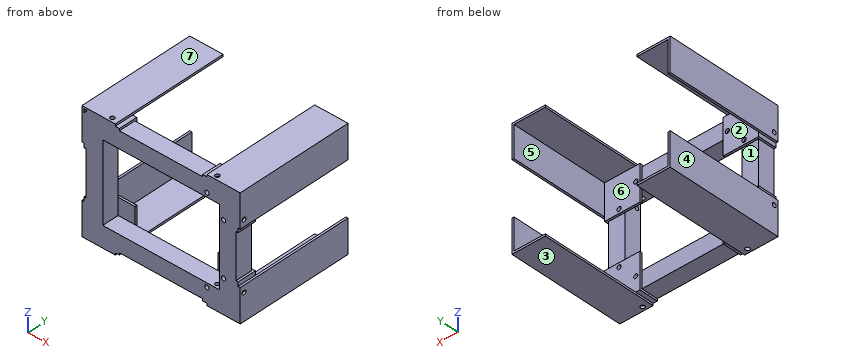
from build123d import *
from build123d.topology import SkipClean

# Parameters (mm, degrees)
SKETCH2_W             = 25.4
SKETCH2_H             = 119.38
BOSS_EXTRUDE1_DEPTH   = 25.4
SKETCH8_W             = 50.8
SKETCH8_H             = 3.175
BOSS_EXTRUDE9_DEPTH   = 25.4
SKETCH11_W            = 53.975
SKETCH11_H            = 53.975
BOSS_EXTRUDE12_DEPTH  = 3.175
CHAMFER3_SIZE         = 5.08
SKETCH10_W            = 3.175
SKETCH10_H            = 47.625
BOSS_EXTRUDE11_DEPTH  = 177.8
SKETCH13_R            = 3.175
CUT_EXTRUDE3_DEPTH    = 31.75
SKETCH14_R            = 3.175
CUT_EXTRUDE4_DEPTH    = 28.575
SKETCH16_R            = 3.175
CUT_EXTRUDE5_DEPTH    = 31.75
MIRROR71_START        = -1
MIRROR71_OUTLINE_R    = 3.175
MIRROR71_DEPTH        = 26.4
MIRROR71_2_DEPTH      = 177.8
MIRROR71_START_2      = 25.4
MIRROR71_3_OUTLINE_R  = 3.175
MIRROR71_3_DEPTH      = 3.175
MIRROR71_START_3      = 9.525
MIRROR71_4_OUTLINE_R  = 3.175
MIRROR71_4_DEPTH      = 15.875
MIRROR71_5_OUTLINE_R  = 3.175
MIRROR71_5_DEPTH      = 3.1749999
MIRROR71_START_4      = 2.6969085
MIRROR71_6_OUTLINE_R  = 3.175
MIRROR71_6_DEPTH      = 17.145
MIRROR71_START_5      = -85.09
MIRROR71_7_OUTLINE_W  = 3.175
MIRROR71_7_OUTLINE_H  = 6.3500001
MIRROR71_7_OUTLINE_R  = 3.175
MIRROR71_7_DEPTH      = 25.4
MIRROR71_START_6      = 59.69
MIRROR71_8_DEPTH      = 28.575
MIRROR71_START_7      = -88.265
MIRROR71_9_DEPTH      = 3.175
MIRROR71_START_8      = 85.09
MIRROR71_10_DEPTH     = 3.175
MIRROR71_START_9      = -91.896565
MIRROR71_11_OUTLINE_W = 6.3500001
MIRROR71_11_OUTLINE_H = 25.4
MIRROR71_11_DEPTH     = 155.396565
MIRROR71_START_10     = 88.9
MIRROR71_12_DEPTH     = 28.575
MIRROR71_START_11     = -114.3
MIRROR71_13_OUTLINE_R = 3.175
MIRROR71_13_DEPTH     = 25.4
MIRROR71_START_12     = 114.3
MIRROR71_14_DEPTH     = 3.175
MIRROR71_START_13     = -92
MIRROR71_15_OUTLINE_R = 3.175
MIRROR71_15_DEPTH     = 184
MIRROR71_16_OUTLINE_R = 3.175
MIRROR71_16_DEPTH     = 33.1


with BuildPart() as part:
    # Sketch2 → Boss-Extrude1 (new body)
    with BuildSketch(Plane(origin=(0, 0, 0), x_dir=(1, 0, 0), z_dir=(0, 1, 0))):
        Polygon((114.3, -59.69), (88.9, -59.69), (-88.9, -59.69), (-114.3, -59.69), (-114.3, -85.09), (114.3, -85.09), align=None)
        with Locations((101.6, 0)):
            Rectangle(SKETCH2_W, SKETCH2_H)
        Polygon((-88.9, 59.69), (88.9, 59.69), (114.3, 59.69), (114.3, 85.09), (-114.3, 85.09), (-114.3, 59.69), align=None)
        with Locations((-101.6, 0)):
            Rectangle(SKETCH2_W, SKETCH2_H)
    boss_extrude1 = extrude(amount=BOSS_EXTRUDE1_DEPTH)

    # Sketch8 → Boss-Extrude9 (add)
    with BuildSketch(Plane(origin=(0, 25.4, 0), x_dir=(1, 0, 0), z_dir=(0, 1, 0))):
        with Locations((-88.9, -86.6775)):
            Rectangle(SKETCH8_W, SKETCH8_H)
        Polygon((-114.3, -88.265), (-114.3, -85.09), (-114.3, -34.29), (-117.475, -34.29), (-117.475, -88.265), align=None)
    boss_extrude9 = extrude(amount=-BOSS_EXTRUDE9_DEPTH)

    # Sketch11 → Boss-Extrude12 (add)
    with BuildSketch(Plane(origin=(0, 25.4, 0), x_dir=(1, 0, 0), z_dir=(0, 1, 0))):
        with Locations((-90.4875, -61.2775)):
            Rectangle(SKETCH11_W, SKETCH11_H)
    boss_extrude12 = extrude(amount=BOSS_EXTRUDE12_DEPTH)

    # Chamfer3
    chamfer3_edges = [part.edges().sort_by_distance(p)[0] for p in [
        (-117.475, 14.2875, 88.265),
    ]]
    chamfer(chamfer3_edges, length=CHAMFER3_SIZE)

    # Sketch10 → Boss-Extrude11 (add)
    with BuildSketch(Plane(origin=(0, 0, 0), x_dir=(-1, 0, 0), z_dir=(0, -1, 0))):
        with Locations((119.0625, -64.4525)):
            Rectangle(SKETCH10_W, SKETCH10_H)
        Polygon((120.65, -88.265), (117.475, -88.265), (69.85, -88.265), (69.85, -91.44), (120.65, -91.44), align=None)
    boss_extrude11 = extrude(amount=-BOSS_EXTRUDE11_DEPTH)

    # Sketch13 → Cut-Extrude3 (cut)
    with BuildSketch(Plane.XY.offset(91.44)):
        with Locations((-80.01, 6.35)):
            Circle(SKETCH13_R)
    cut_extrude3 = extrude(amount=-CUT_EXTRUDE3_DEPTH, mode=Mode.SUBTRACT)

    # Sketch14 → Cut-Extrude4 (cut)
    with BuildSketch(Plane(origin=(0, 28.575, 0), x_dir=(1, 0, 0), z_dir=(0, 1, 0))):
        with Locations(Location((-69.85, -66.04, 0), (0, 0, 270))):
            Circle(SKETCH14_R)
        with Locations(Location((-95.25, -40.64, 0), (0, 0, 270))):
            Circle(SKETCH14_R)
    cut_extrude4 = extrude(amount=-CUT_EXTRUDE4_DEPTH, mode=Mode.SUBTRACT)

    # Sketch16 → Cut-Extrude5 (cut)
    with BuildSketch(Plane.ZY.offset(120.65)):
        with Locations((50.8, 6.35)):
            Circle(SKETCH16_R)
    cut_extrude5 = extrude(amount=-CUT_EXTRUDE5_DEPTH, mode=Mode.SUBTRACT)

    # Mirror70: Boss-Extrude1, Boss-Extrude9, Boss-Extrude12, Boss-Extrude11, Cut-Extrude3, Cut-Extrude4, Cut-Extrude5 across plane
    add(boss_extrude1.mirror(Plane.XY))
    add(boss_extrude9.mirror(Plane.XY))
    add(boss_extrude12.mirror(Plane.XY))
    add(boss_extrude11.mirror(Plane.XY))
    add(cut_extrude3.mirror(Plane.XY), mode=Mode.SUBTRACT)
    add(cut_extrude4.mirror(Plane.XY), mode=Mode.SUBTRACT)
    add(cut_extrude5.mirror(Plane.XY), mode=Mode.SUBTRACT)

    # Mirror71: read off the stored shape, not the designer's step
    # Mirror71 outline → Mirror71 (cut)
    with BuildSketch(Plane(origin=(0, 0, 0), x_dir=(1, 0, 0), z_dir=(0, 1, 0)).offset(MIRROR71_START)):
        with Locations((69.85, 66.04)):
            Circle(MIRROR71_OUTLINE_R)
        with Locations((95.25, 40.64)):
            Circle(MIRROR71_OUTLINE_R)
        with Locations((69.85, -66.04)):
            Circle(MIRROR71_OUTLINE_R)
        with Locations((95.25, -40.64)):
            Circle(MIRROR71_OUTLINE_R)
    extrude(amount=MIRROR71_DEPTH, mode=Mode.SUBTRACT)



with BuildPart() as body_2:
    # Mirror71 2 outline → Mirror71 2 (new body)
    with BuildSketch(Plane(origin=(0, 0, 0), x_dir=(1, 0, 0), z_dir=(0, 1, 0))):
        Polygon((117.475, -88.265), (69.85, -88.265), (69.85, -91.44), (120.65, -91.44), (120.65, -40.64), (117.475, -40.64), align=None)
        Polygon((117.475, 88.265), (117.475, 40.64), (120.65, 40.64), (120.65, 91.44), (69.85, 91.44), (69.85, 88.265), align=None)
    extrude(amount=MIRROR71_2_DEPTH)


with BuildPart() as part_1:
    add(part.part)

    add(body_2.part)  # Mirror71 3 merges body 2
    # Mirror71 3 outline → Mirror71 3 (add)
    # profile 1 of 2: a face of its own
    with BuildSketch(Plane(origin=(0, 0, 0), x_dir=(1, 0, 0), z_dir=(0, 1, 0)).offset(MIRROR71_START_2)):
        Polygon((63.5, -88.265), (117.475, -88.265), (117.475, -34.29), (88.9, -34.29), (63.5, -34.29), align=None)
        with Locations((95.25, -40.64)):
            Circle(MIRROR71_3_OUTLINE_R, mode=Mode.SUBTRACT)
        with Locations((69.85, -66.04)):
            Circle(MIRROR71_3_OUTLINE_R, mode=Mode.SUBTRACT)
    # profile 2 of 2: a face of its own
    with BuildSketch(Plane(origin=(0, 0, 0), x_dir=(1, 0, 0), z_dir=(0, 1, 0)).offset(MIRROR71_START_2)):
        Polygon((63.5, 34.29), (88.9, 34.29), (117.475, 34.29), (117.475, 88.265), (63.5, 88.265), align=None)
        with Locations((95.25, 40.64)):
            Circle(MIRROR71_3_OUTLINE_R, mode=Mode.SUBTRACT)
        with Locations((69.85, 66.04)):
            Circle(MIRROR71_3_OUTLINE_R, mode=Mode.SUBTRACT)
    extrude(amount=MIRROR71_3_DEPTH)

    # Mirror71 4 outline → Mirror71 4 (add)
    with BuildSketch(Plane(origin=(0, 0, 0), x_dir=(1, 0, 0), z_dir=(0, 1, 0)).offset(MIRROR71_START_3)):
        Polygon((63.5, -88.265), (117.475, -88.265), (117.475, -34.29), (114.3, -34.29), (114.3, -85.09), (63.5, -85.09), align=None)
        Polygon((114.3, 85.09), (114.3, 34.29), (117.475, 34.29), (117.475, 88.265), (63.5, 88.265), (63.5, 85.09), align=None)
        with Locations((-69.85, 66.04)):
            Circle(MIRROR71_4_OUTLINE_R)
        with Locations((-95.25, 40.64)):
            Circle(MIRROR71_4_OUTLINE_R)
    extrude(amount=MIRROR71_4_DEPTH)

    # Mirror71 5 outline → Mirror71 5 (add)
    with BuildSketch(Plane(origin=(0, 0, 0), x_dir=(1, 0, 0), z_dir=(0, 1, 0))):
        Polygon((63.5, -88.265), (117.475, -88.265), (117.475, -34.29), (114.3, -34.29), (114.3, -85.09), (63.5, -85.09), align=None)
        Polygon((114.3, 85.09), (114.3, 34.29), (117.475, 34.29), (117.475, 88.265), (63.5, 88.265), (63.5, 85.09), align=None)
        with Locations((-69.85, 66.04)):
            Circle(MIRROR71_5_OUTLINE_R)
        with Locations((-95.25, 40.64)):
            Circle(MIRROR71_5_OUTLINE_R)
    extrude(amount=MIRROR71_5_DEPTH)

    # Mirror71 6 outline → Mirror71 6 (add)
    with BuildSketch(Plane(origin=(0, 0, 0), x_dir=(1, 0, 0), z_dir=(0, 1, 0)).offset(MIRROR71_START_4)):
        with Locations((-69.85, 66.04)):
            Circle(MIRROR71_6_OUTLINE_R)
        with Locations((-95.25, 40.64)):
            Circle(MIRROR71_6_OUTLINE_R)
    extrude(amount=MIRROR71_6_DEPTH)

    # Mirror71 7 outline → Mirror71 7 (add)
    with BuildSketch(Plane.XY.offset(MIRROR71_START_5)):
        with Locations((115.8875, 6.34999995)):
            Rectangle(MIRROR71_7_OUTLINE_W, MIRROR71_7_OUTLINE_H)
        with Locations((-80.01, 6.35)):
            Circle(MIRROR71_7_OUTLINE_R)
    extrude(amount=MIRROR71_7_DEPTH)

    # Mirror71 8 outline → Mirror71 8 (add)
    with BuildSketch(Plane.XY.offset(MIRROR71_START_6)):
        with BuildLine():
            ThreePointArc((80.01, 9.525), (83.185, 6.35), (80.01, 3.175))
            Line((80.01, 3.175), (117.475, 3.1749999))
            Line((117.475, 3.1749999), (117.475, 9.525))
            Line((117.475, 9.525), (80.01, 9.525))
        make_face()
    extrude(amount=MIRROR71_8_DEPTH)

    # Mirror71 9 outline → Mirror71 9 (add)
    with BuildSketch(Plane.XY.offset(MIRROR71_START_7)):
        with BuildLine():
            ThreePointArc((80.01, 9.525), (83.185, 6.35), (80.01, 3.175))
            Line((80.01, 3.175), (117.475, 3.1749999))
            Line((117.475, 3.1749999), (117.475, 9.525))
            Line((117.475, 9.525), (80.01, 9.525))
        make_face()
        with BuildLine():
            ThreePointArc((80.01, 3.175), (76.835, 6.35), (80.01, 9.525))
            Line((80.01, 9.525), (63.5, 9.525))
            Line((63.5, 9.525), (63.5, 3.1749999))
            Line((63.5, 3.1749999), (80.01, 3.175))
        make_face()
    extrude(amount=MIRROR71_9_DEPTH)

    # Mirror71 10 outline → Mirror71 10 (add)
    with BuildSketch(Plane.XY.offset(MIRROR71_START_8)):
        with BuildLine():
            ThreePointArc((80.01, 3.175), (76.835, 6.35), (80.01, 9.525))
            Line((80.01, 9.525), (63.5, 9.525))
            Line((63.5, 9.525), (63.5, 3.1749999))
            Line((63.5, 3.1749999), (80.01, 3.175))
        make_face()
    extrude(amount=MIRROR71_10_DEPTH)

    # Mirror71 11 outline → Mirror71 11 (add)
    with BuildSketch(Plane.YZ.offset(MIRROR71_START_9)):
        with Locations((6.34999995, -72.39)):
            Rectangle(MIRROR71_11_OUTLINE_W, MIRROR71_11_OUTLINE_H)
    extrude(amount=MIRROR71_11_DEPTH)

    # Mirror71 12 outline → Mirror71 12 (add)
    with BuildSketch(Plane.YZ.offset(MIRROR71_START_10)):
        with BuildLine():
            ThreePointArc((9.525, -50.8), (6.35, -53.975), (3.175, -50.8))
            Line((3.175, -50.8), (3.1749999, -88.265))
            Line((3.1749999, -88.265), (9.525, -88.265))
            Line((9.525, -88.265), (9.525, -50.8))
        make_face()
        with BuildLine():
            ThreePointArc((3.175, 50.8), (6.35, 53.975), (9.525, 50.8))
            Line((9.525, 50.8), (9.525, 88.265))
            Line((9.525, 88.265), (3.1749999, 88.265))
            Line((3.1749999, 88.265), (3.175, 50.8))
        make_face()
    extrude(amount=MIRROR71_12_DEPTH)

    # Mirror71 13 outline → Mirror71 13 (add)
    with BuildSketch(Plane.YZ.offset(MIRROR71_START_11)):
        with Locations((6.35, -50.8)):
            Circle(MIRROR71_13_OUTLINE_R)
    extrude(amount=MIRROR71_13_DEPTH)

    # Mirror71 14 outline → Mirror71 14 (add)
    with BuildSketch(Plane.YZ.offset(MIRROR71_START_12)):
        with BuildLine():
            ThreePointArc((3.175, -50.8), (6.35, -47.625), (9.525, -50.8))
            Line((9.525, -50.8), (9.525, -34.29))
            Line((9.525, -34.29), (3.1749999, -34.29))
            Line((3.1749999, -34.29), (3.175, -50.8))
        make_face()
        with BuildLine():
            Line((9.525, 34.29), (9.525, 50.8))
            ThreePointArc((9.525, 50.8), (6.35, 47.625), (3.175, 50.8))
            Line((3.175, 50.8), (3.1749999, 34.29))
            Line((3.1749999, 34.29), (9.525, 34.29))
        make_face()
    extrude(amount=MIRROR71_14_DEPTH)

    # Mirror71 15 outline → Mirror71 15 (cut)
    with SkipClean():  # the faces are left unmerged after this step: merging them gives an invalid solid
        with BuildSketch(Plane.XY.offset(MIRROR71_START_13)):
            with Locations((80.01, 6.35)):
                Circle(MIRROR71_15_OUTLINE_R)
        extrude(amount=MIRROR71_15_DEPTH, mode=Mode.SUBTRACT)

    # Mirror71 16 outline → Mirror71 16 (cut)
    with SkipClean():  # the faces are left unmerged after this step: merging them gives an invalid solid
        with BuildSketch(Plane.YZ.offset(MIRROR71_START_10)):
            with Locations((6.35, -50.8)):
                Circle(MIRROR71_16_OUTLINE_R)
            with Locations((6.35, 50.8)):
                Circle(MIRROR71_16_OUTLINE_R)
        extrude(amount=MIRROR71_16_DEPTH, mode=Mode.SUBTRACT)


solid = part_1.part
For this review, take the finished solid that the model builds, in its own axes (mm). Face numbers are marked on the shaded views. A direction names the side the tool comes from. Give positions to 0.01 mm unless a question says otherwise; leave off trailing zeros. Loops run counter-clockwise (first coordinate to the right, second up) from the corner with the lowest first, then second, coordinate; pieces in that order, holes last.
Item 1: Take a section at B-B, the plane y = 56. State the section outline as (x, z) points (3 decimals).
Item 2: Take a section at D-D, the plane x = -95.25. State the section outline as (y, z) points (3 decimals).
Item 3: Take a section at C-C, the plane z = -27. State the section outline as (x, y) points, and give its area (3 significant figures).
Item 4: Draft analysis for pull direction X (two halves, no side actions). For the marked faces 4, 5, 6 and 7, state which applies: +X half, -X half, draft (parallel to the pull), parting line (faces both ways), or undercut.
Item 5: Tool access review of the marked faces 1, 2 and 3: name each direction out of +Z, -Z, +X, -X, +Y, -Y from which nothing blocks a thin tool from reaching the whole face with its end or side.
Item 6: Take a section at A-A, the plane x = 53.5. State the section outline as (y, z) points.
Item 7: Insertion check: pin 1 (7.5 mm diameter, centred on x = -31, y = 13, fed in from -Z); pin 2 (7.5 mm diameter, centred on x = -70.5, z = -42, fed in from -Y); pin 3 (10 mm diameter, centred on x = 95.25, z = 40.64, fed in from +Y) (3 decimals); pin 4 (12 mm diameter, centred on y = 83, z = -31, fed in from -X). Each pin has a flat end and moves straight along its axis. Give the tip position at first contact, or say it passes through.
Item 8: For line 1 along X through (y, z) = (150.5, 68) (3 decimals); line 2 along Y through (x, z) = (80, -87) (3 decimals); line 3 along Y through (x, z) = (-80.01, 89.5) (3 decimals), list the stretches that pass through material, from the lowest coordinate up.
Calculated:
1. outline: (-120.65, -91.44) - (-69.85, -91.44) - (-69.85, -88.265) - (-117.475, -88.265) - (-117.475, -40.64) - (-120.65, -40.64) - close; (-120.65, 40.64) - (-117.475, 40.64) - (-117.475, 88.265) - (-69.85, 88.265) - (-69.85, 91.44) - (-120.65, 91.44) - close; (69.85, -91.44) - (120.65, -91.44) - (120.65, -40.64) - (117.475, -40.64) - (117.475, -88.265) - (69.85, -88.265) - close; (69.85, 88.265) - (117.475, 88.265) - (117.475, 40.64) - (120.65, 40.64) - (120.65, 91.44) - (69.85, 91.44) - close
2. outline: (0, -91.44) - (177.8, -91.44) - (177.8, -88.265) - (28.575, -88.265) - (28.575, -43.815) - (25.4, -43.815) - (25.4, -37.465) - (28.575, -37.465) - (28.575, -34.29) - (25.4, -34.29) - (25.4, 34.29) - (28.575, 34.29) - (28.575, 37.465) - (25.4, 37.465) - (25.4, 43.815) - (28.575, 43.815) - (28.575, 88.265) - (177.8, 88.265) - (177.8, 91.44) - (0, 91.44) - close
3. outline: (-114.3, 0) - (-88.9, 0) - (-88.9, 25.4) - (-114.3, 25.4) - close; (88.9, 0) - (114.3, 0) - (114.3, 25.4) - (88.9, 25.4) - close
3. area: 1,290 mm2
4. face 4: -X half
4. face 5: undercut
4. face 6: undercut
4. face 7: draft
5. face 1: +X, -X, +Y
5. face 2: +Y
5. face 3: -Z, +X, -X, +Y, -Y
6. outline: (0, -85.09) - (25.4, -85.09) - (25.4, -59.69) - (0, -59.69) - close; (0, 59.69) - (25.4, 59.69) - (25.4, 85.09) - (0, 85.09) - close
7. pin 1: stops at z = -85.09
7. pin 2: stops at y = 25.4
7. pin 3: stops at y = 28.575
7. pin 4: passes through
8. line 1: x = -120.65 to -117.475, 117.475 to 120.65
8. line 2: y = 0 to 3.175, 9.525 to 28.575
8. line 3: y = 0 to 3.175, 9.525 to 177.8
